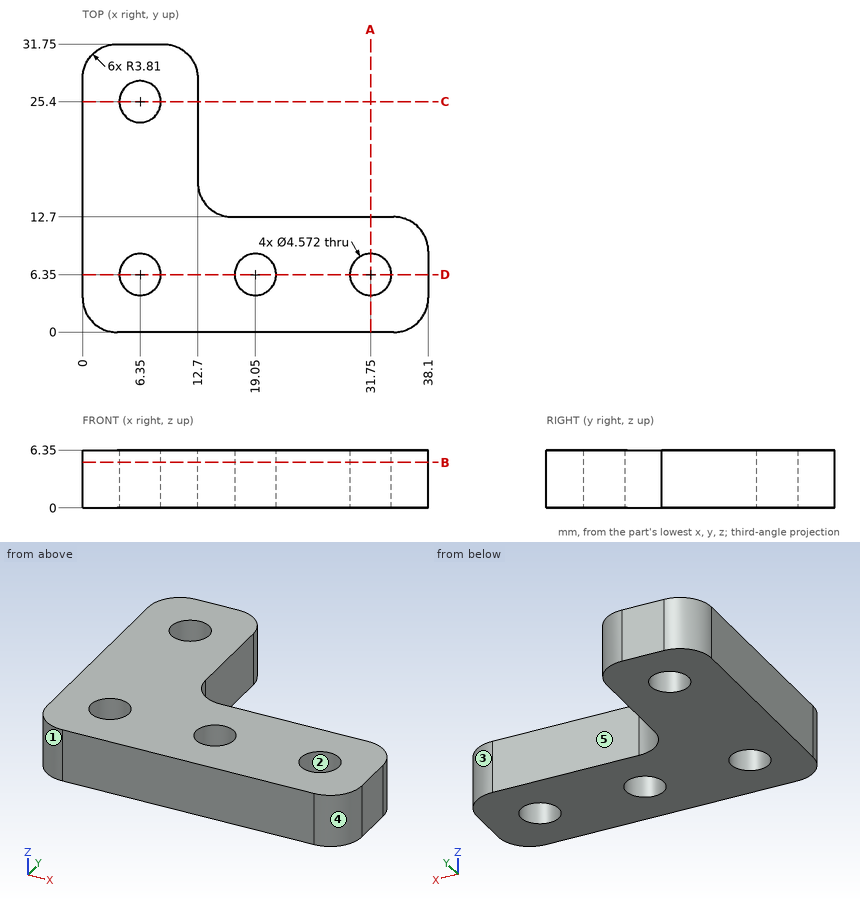
The figure shows three views and two pictorial views of one solid part (mm, origin at its lowest corner). Answer the questions. A direction names the side the tool comes from. Coordinates: 2 decimals unless noted, no trailing zeros. Loops run counter-clockwise (first coordinate to the right, second up) from the corner with the lowest first, then second, coordinate; pieces in that order, holes last. Notation, with made-up numbers: (82.25, -36) -> (102.25, -36) arc R28 ccw to (102.25, 0) -> close; hole circle Ø9 at (57, -18). An arc over 180 degrees is marked (long way). Use one line per item in the form item = value. Start each with the question number.
Item 1: The part is cut by section B-B on z = 5. Determine the outline of the cut face in (x, y).
Item 2: Flat-ended cylindrical pins translate along their axes: pin 1 Ø1.9 at (x, z) = (21, 1.5) entering from +Y; pin 2 Ø1.9 at (y, z) = (23.5, 3) entering from +X. Find the tip coordinate at first contact, or state that the pin passes through.
Item 3: A tool of negligible diameter and unlimited length cuts with its end or side. For the marked faces 4 and 5, from which of +Z, -Z, +X, -X, +Y, -Y can it reach the whole face along a straight path? Write none if from no direction.
Item 4: The part is cut by section A-A on x = 31.75. Determine the outline of the cut face in (y, z), then the cut area to 3 significant figures.
Item 5: The mould has two halves that part along X. Classify the marked faces 1, 2 and 3: released by +X, released by -X, zero draft, split by the parting line, or undercut.
Item 6: The part is cut by section D-D on y = 6.35. Determine the outline of the cut face in (x, z), then the cut area to 3 significant figures.
Item 7: Consider L1, parallel to X at y = 6.5, z = 3; L2, parallel to X at y = 4.5, z = 3.75; L3, parallel to Y at x = 5, z = 2. Determine where each line is inside the solid, lowest interval first. Write a range as [from, to].
Answer key:
q1.outline = (0, 3.81) arc R3.81 ccw to (3.81, 0) -> (34.29, 0) arc R3.81 ccw to (38.1, 3.81) -> (38.1, 8.89) arc R3.81 ccw to (34.29, 12.7) -> (16.51, 12.7) arc R3.81 cw to (12.7, 16.51) -> (12.7, 27.94) arc R3.81 ccw to (8.89, 31.75) -> (3.81, 31.75) arc R3.81 ccw to (0, 27.94) -> close; hole circle Ø4.57 at (6.35, 6.35); hole circle Ø4.57 at (6.35, 25.4); hole circle Ø4.57 at (19.05, 6.35); hole circle Ø4.57 at (31.75, 6.35)
q2.pin_1 = 12.7
q2.pin_2 = 12.7
q3.face_4 = +Z, -Z, +X, -Y
q3.face_5 = +Z, -Z, +X, +Y
q4.outline = (0, 0) -> (4.06, 0) -> (4.06, 6.35) -> (0, 6.35) -> close; (8.64, 0) -> (12.7, 0) -> (12.7, 6.35) -> (8.64, 6.35) -> close
q4.area = 51.6 mm2
q5.face_1 = released by -X
q5.face_2 = undercut
q5.face_3 = released by +X
q6.outline = (0, 0) -> (4.06, 0) -> (4.06, 6.35) -> (0, 6.35) -> close; (8.64, 0) -> (16.76, 0) -> (16.76, 6.35) -> (8.64, 6.35) -> close; (21.34, 0) -> (29.46, 0) -> (29.46, 6.35) -> (21.34, 6.35) -> close; (34.04, 0) -> (38.1, 0) -> (38.1, 6.35) -> (34.04, 6.35) -> close
q6.area = 155 mm2
q7.L1 = [0, 4.07], [8.63, 16.77], [21.33, 29.47], [34.03, 38.1]
q7.L2 = [0, 5.01], [7.69, 17.71], [20.39, 30.41], [33.09, 38.1]
q7.L3 = [0, 4.51], [8.19, 23.56], [27.24, 31.75]
